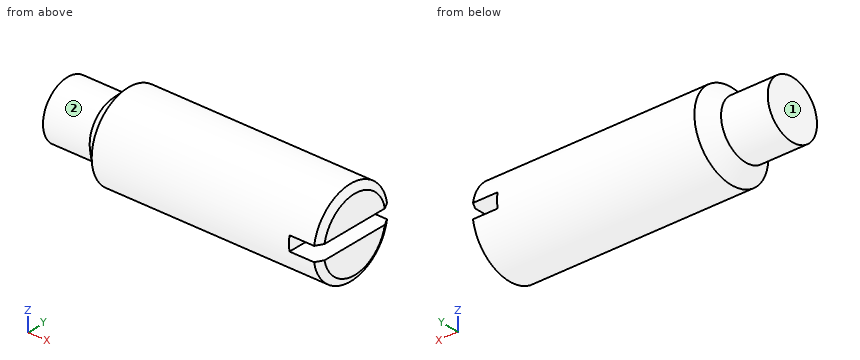
from build123d import *

# Parameters (mm, degrees)
CHAMFER1_SIZE      = 0.5
CHAMFER1_SIZE2     = 0.288675135
SKETCH2_W          = 1
SKETCH2_H          = 6
CUT_EXTRUDE2_DEPTH = 2


with BuildPart() as part:
    # Sketch1 → Revolve1 (revolve)
    with BuildSketch(Plane.XY, mode=Mode.PRIVATE) as revolve1_sk:
        Polygon((0, 0), (0, 3), (-15.75, 3), (-16.75, 2), (-20, 2), (-20, 0), align=None)
    revolve(revolve1_sk.sketch.rotate(Axis((-20, 0, 0), (1, 0, 0)), 180), axis=Axis((-20, 0, 0), (1, 0, 0)))

    # Chamfer1
    chamfer1_edges = [part.edges().sort_by_distance(p)[0] for p in [
        (0, 3, 0),
    ]]
    chamfer1_side = [part.faces().sort_by_distance(p)[0] for p in [
        (0, 0, 0),
    ]]
    chamfer(chamfer1_edges, length=CHAMFER1_SIZE, length2=CHAMFER1_SIZE2, reference=chamfer1_side[0])

    # Sketch2 → Cut-Extrude2 (cut)
    with BuildSketch(Plane(origin=(0, 0, 0), x_dir=(0, 0, -1), z_dir=(1, 0, 0))):
        Rectangle(SKETCH2_W, SKETCH2_H)
    extrude(amount=-CUT_EXTRUDE2_DEPTH, mode=Mode.SUBTRACT)


solid = part.part
Design review of the part built by this model. Coordinates are the model's own, in mm. Face numbers are marked on the shaded views. A direction names the side the tool comes from. Round coordinates to 2 decimals unless told otherwise and drop trailing zeros. Loops run counter-clockwise (first coordinate to the right, second up) from the corner with the lowest first, then second, coordinate; pieces in that order, holes last. Notation, with made-up numbers: M 42.5,-9.75 L 92.5,-9.75 A17 cw 92.5,14.25 Z; hole C 6,61.25 d9. An arc over 180 degrees is marked long. Answer as a JSON object with one key per item and string values.
Item 1: We need section B-B on z = 0. Give the boundary of the cut face in (x, y), and give its area (4 significant figures).
Answer sheet:
{"outline": "M -20,-2 L -16.75,-2 L -15.75,-3 L -2,-3 L -2,3 L -15.75,3 L -16.75,2 L -20,2 Z", "area": "100.5 mm^2"}
Item 2: We need section A-A on y = 0. Give the boundary of the cut face in (x, z).
Answer sheet:
{"outline": "M -20,-2 L -16.75,-2 L -15.75,-3 L -0.29,-3 L 0,-2.5 L 0,-0.5 L -2,-0.5 L -2,0.5 L 0,0.5 L 0,2.5 L -0.29,3 L -15.75,3 L -16.75,2 L -20,2 Z"}
Item 3: Clearance check with flat-ended pins moving along their axes: P1, Ø1, axis at x = -1.5, y = -1, coming from the +Z side; P2, Ø0.6, axis at x = -0.5, y = 0.5, coming from the -Z side; P3, Ø2, axis at x = -16.5, z = 2.5, coming from the +Y side. State where each tip first meets the part, or that it passes through.
Answer sheet:
{"P1": "stops at z = 2.96", "P2": "stops at z = -2.99", "P3": "stops at y = 2.37"}
Item 4: Wall thickness on L1, parallel to Z at x = -19, y = 0; L2, parallel to Z at x = -1.5, y = -1.5; L3, parallel to Z at x = -1.5, y = 2.55: over which ranges is each line inside the solid? List them lowest first. Write a range as from..to.
Answer sheet:
{"L1": "z = -2..2", "L2": "z = -2.6..-0.5, 0.5..2.6", "L3": "z = -1.58..-0.5, 0.5..1.58"}
Item 5: We need section C-C on x = -3.5. Give the boundary of the cut face in (y, z).
Answer sheet:
{"outline": "C 0,0 d6"}
Item 6: Machinability: for the marked faces 1 and 2, which of the approach directions +Z, -Z, +X, -X, +Y, -Y give a long, thin tool a straight path to every point of the face, cutting with its end or side? Answer none if there is none.
Answer sheet:
{"face 1": "+Z, -Z, -X, +Y, -Y", "face 2": "-X"}
Item 7: We need section D-D on x = -16.5. Give the boundary of the cut face in (y, z), and give its area (3 significant figures).
Answer sheet:
{"outline": "C 0,0 d4.5", "area": "15.9 mm^2"}
